Design review of the part built by this model. Coordinates are the model's own, in mm. A direction names the side the tool comes from. Give positions to 0.01 mm unless a question says otherwise; leave off trailing zeros. Order: outer loops, then holes, each group sorted by start corner. A loop starts at its lowest first (then second) coordinate and runs counter-clockwise, first axis right, second up.
Autodesk Inventor part; units mm, degrees
ref_plane "YZ Plane" through (0, 0, 0) normal (1, 0, 0) x (0, 1, 0)
ref_plane "XZ Plane" through (0, 0, 0) normal (0, 1, 0) x (-1, 0, 0)
ref_plane "XY Plane" through (0, 0, 0) normal (0, 0, 1) x (1, 0, 0)
sketch "Sketch1" plane through (0, 0, 0) normal (0, 1, 0) x (-1, 0, 0)
  line L0 (0, 0) -> (-50.8, 0)
  line L1 (-50.8, 0) -> (-50.8, 1016)
  line L2 (-50.8, 1016) -> (0, 1016)
  line L3 (0, 1016) -> (0, 0)
  dimension "d0" = 1016
  dimension "d1" = 50.8
extrude "Extrusion1" add sketch "Sketch1" along normal blind 25.4
sketch "Sketch2" plane through (0, 0, 0) normal (0, -1, 0) x (1, 0, 0)
  line L0 (0, 838.2) -> (50.8, 838.2)
  line L1 (50.8, 838.2) -> (50.8, 863.6)
  line L2 (50.8, 863.6) -> (0, 863.6)
  line L3 (0, 863.6) -> (0, 838.2)
  line L4 (50.8, 1016) -> (0, 1016)
  line L5 (50.8, 0) -> (0, 0)
  line L6 (50.8, 0) -> (0, 0)
  line L7 (0, 0) -> (0, 25.4)
  line L8 (0, 25.4) -> (50.8, 25.4)
  line L9 (50.8, 25.4) -> (50.8, 0)
  dimension "d4" = 25.4
  dimension "d7" = 152.4
  dimension "d30" = 25.4
extrude "Extrusion2" add sketch "Sketch2" along normal blind 279.4
sketch "Sketch3" plane through (0, -279.4, 0) normal (0, -1, 0) x (1, 0, 0)
  line L0 (50.8, 0) -> (0, 0)
  line L1 (0, 1016) -> (50.8, 1016)
  line L2 (0, 0) -> (50.8, 0)
  line L3 (50.8, 0) -> (50.8, 1016)
  line L4 (50.8, 1016) -> (0, 1016)
  line L5 (0, 1016) -> (0, 0)
extrude "Extrusion3" add sketch "Sketch3" along normal blind 25.4
sketch "Sketch4" plane through (0, -279.4, 0) normal (0, 1, 0) x (1, 0, 0)
  circle A0 centre (25.4, -635) radius 12.7
  line L0 (0, -1016) -> (50.8, -1016)
  line L1 (0, -1016) -> (0, -863.6)
  point P0 (0, 0)
  dimension "d12" = 25.4
  dimension "d13" = 381
  dimension "d18" = 25.4
extrude "Extrusion4" add sketch "Sketch4" along normal blind 284.1625
properties part number "stage"
1. Take a section at C-C (x = 25.4). State the section outline as (y, z) points, then the cut area to 3 significant figures.
Recorded:
outline: (-304.8, 0) - (25.4, 0) - (25.4, 1016) - (0, 1016) - (0, 863.6) - (-279.4, 863.6) - (-279.4, 1016) - (-304.8, 1016) - close; hole (-279.4, 25.4) - (0, 25.4) - (0, 622.3) - (-279.4, 622.3) - close; hole (-279.4, 647.7) - (0, 647.7) - (0, 838.2) - (-279.4, 838.2) - close
area: 72,900 mm2
2. For line 1 along Z through (x, y) = (26, -92); line 2 along Z through (x, y) = (11.5, -198.5); line 3 along Y through (x, z) = (27.5, 935), list the stretches that pass through material, from the lowest coordinate up.
Recorded:
line 1: z = 0 to 25.4, 622.31 to 647.69, 838.2 to 863.6
line 2: z = 0 to 25.4, 838.2 to 863.6
line 3: y = -304.8 to -279.4, 0 to 25.4
3. Draft analysis for pull direction Z (two halves, no side actions). For faces 4 (the face through (26, -137, 0)), 5 (the face through (23.747, -141.656, 647.592)), 6 (the face through (26, -138, 863.6)), state which applies: pulls with the +Z half, pulls with the -Z half, needs draft (parallel to the pull), parting line crosses it, or undercut.
Recorded:
face 4: pulls with the -Z half
face 5: undercut
face 6: pulls with the +Z half
4. Take a section at A-A (z = 900). State the section outline as (x, y) points.
Recorded:
outline: (0, -304.8) - (50.8, -304.8) - (50.8, -279.4) - (0, -279.4) - close; (0, 0) - (50.8, 0) - (50.8, 25.4) - (0, 25.4) - close
5. Take a section at B-B (y = -233). State the section outline as (x, z) points.
Recorded:
outline: (0, 0) - (50.8, 0) - (50.8, 25.4) - (0, 25.4) - close; (0, 838.2) - (50.8, 838.2) - (50.8, 863.6) - (0, 863.6) - close; circle Ø25.4 at (25.4, 635)
6. For pin 1 (8 mm diameter, centred on x = 44, y = -167.5, fed in from +Z), flat-tipped, find the tip position at first contact; note if it passes through.
Recorded:
pin 1: stops at z = 863.6
7. Machinability: for faces 1 (the face through (25, -138, 25.4)), 2 (the face through (26, 0, 941)), 3 (the face through (50.8, -286, 468)), which of the approach directions +Z, -Z, +X, -X, +Y, -Y give a long, thin tool a straight path to every point of the face, cutting with its end or side? Answer none if there is none.
Recorded:
face 1: +X, -X
face 2: +Z, +X, -X
face 3: +Z, -Z, +X, +Y, -Y
8. Take a section at D-D (z = 635). State the section outline as (x, y) points, then the cut area to 3 significant figures.
Recorded:
outline: (0, -304.8) - (50.8, -304.8) - (50.8, -279.4) - (38.1, -279.4) - (38.1, 0) - (50.8, 0) - (50.8, 25.4) - (0, 25.4) - (0, 0) - (12.7, 0) - (12.7, -279.4) - (0, -279.4) - close
area: 9,680 mm2
